Read the model definition and answer for the solid it produces. Units are mm, in the model's axes. Coordinates: 2 decimals unless noted, no trailing zeros. Loops run counter-clockwise (first coordinate to the right, second up) from the corner with the lowest first, then second, coordinate; pieces in that order, holes last.
from build123d import *

# Parameters (mm, degrees)
F1_DEPTH = 25.4
F2_DEPTH = 25.4
F3_COUNT = 2
F3_ANGLE = 90
F4_COUNT = 2
F4_ANGLE = 90


with BuildPart() as f1:
    # F0 (on Top) → F1 (new body)
    with BuildSketch(Plane.XY):
        Polygon((-23.5681033644, -10.4691434878), (-8.8881384679, -1.757956216), (-21.7093285173, 9.5116151497), (-32.4273278005, -2.6820611935), align=None)
        Polygon((-8.8881384679, -1.757956216), (-3.2808908311, 1.5694212395), (-8.4611528206, 24.5838280055), (-21.7093285173, 9.5116151497), align=None)
        Polygon((-32.4273278005, -2.6820611935), (-21.7093285173, 9.5116151497), (-34.5305185668, 20.7811865153), (-41.2865522365, 5.1050211008), align=None)
        Polygon((-21.7093285173, 9.5116151497), (-8.4611528206, 24.5838280055), (-31.9499433341, 26.7689488904), (-34.5305185668, 20.7811865153), align=None)
    extrude(amount=-F1_DEPTH)

    # F2 (add): a face of the model
    f2_faces = [f1.faces().sort_by_distance(p)[0] for p in [
        (-21.7093285173, 9.5116151497, 0),
    ]]
    extrude(f2_faces, amount=F2_DEPTH)


with BuildPart() as f3_1:
    # F3: instance of F1
    add(f1.part.rotate(Axis((-20.8140740816, 10.5301301305, 0), (0.6601960829, 0.7510932913, 0)), 1 * F3_ANGLE / (F3_COUNT - 1)))


with BuildPart() as f4_1:
    # F4: instance of F1
    add(f1.part.rotate(Axis((-21.7093285173, 9.5116151497, 0), (0.7510932913, -0.6601960829, 0)), 1 * F4_ANGLE / (F4_COUNT - 1)))


with BuildPart() as f3_1_1:
    add(f3_1.part)

    # F5: intersect F4_1, F1
    add(f4_1.part, mode=Mode.INTERSECT)
    add(f1.part, mode=Mode.INTERSECT)


solid = f3_1_1.part
Q1. A cutting plane is placed at B-B (y = -2.5). Give the vertices of the cut face in (x, z), then the cut area to 3 significant figures.
Findings below:
outline: (-32.63, -11.8) - (-16.17, -15.33) - (-10.14, -1.38) - (-10.14, 7.99) - (-21.49, 14.19) - (-32.63, 11.8) - close
area: 544 mm2
Q2. A cutting plane is placed at D-D (y = 22.5). Give the vertices of the cut face in (x, z).
Findings below:
outline: (-33.79, 1.78) - (-26, -16.23) - (-23.96, -16.23) - (-7.99, -1.73) - (-7.99, 1.73) - (-21.46, 13.97) - (-33.79, 7.24) - close
Q3. A cutting plane is placed at C-C (x = -17.5). Give the vertices of the cut face in (y, z).
Findings below:
outline: (-6.87, -9.52) - (-4.38, -14.58) - (2.39, -16.23) - (16.82, -16.23) - (25.42, -7.34) - (25.42, 7.34) - (14.07, 19.08) - (10.37, 18.18) - (-6.87, 9.91) - close
Q4. A cutting plane is placed at A-A (z = -4). Give the vertices of the cut face in (x, y).
Findings below:
outline: (-41.29, 5.11) - (-23.57, -10.47) - (-12.51, -3.9) - (-4.18, 5.57) - (-7.38, 19.76) - (-13.38, 25.04) - (-27.87, 26.39) - (-36.2, 16.92) - close
Q5. Straight lines are drawn through the part: probe 1 along X at (y, z) = (24, 12); probe 2 along Y at (x, z) = (-22, -8.5); probe 3 along X at (y, z) = (21, -15). For each, find the intervals that lie inside material, in ascending order.
Findings below:
probe 1: x = -23.76 to -21
probe 2: y = -9.54 to 25.84
probe 3: x = -27.85 to -20.89
Q6. Flat-ended cylindrical pins translate along their axes: pin 1 Ø5 at (x, z) = (-8.5, -3.5) entering from +Y; pin 2 Ø1 at (x, y) = (-18.5, -0.5) entering from -Z; pin 3 Ø4 at (y, z) = (10.5, 7.5) entering from +X. Find the tip coordinate at first contact, or state that the pin passes through.
Findings below:
pin 1: stops at y = 24.5
pin 2: stops at z = -15.48
pin 3: stops at x = -4.84
